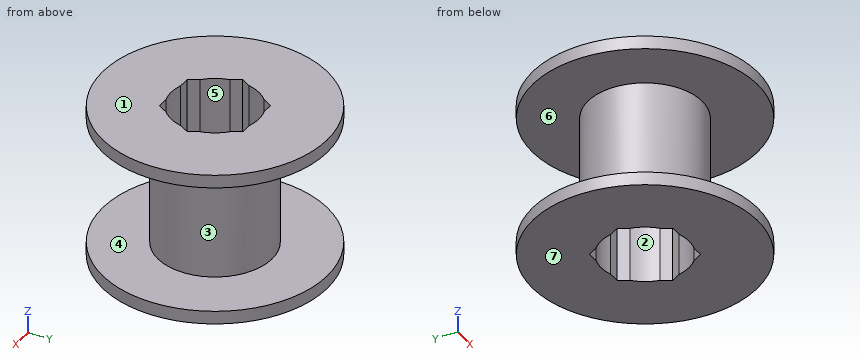
```python
from build123d import *

# Parameters (mm, degrees)
CUT_EXTRUDE1_DEPTH = 33.8


with BuildPart() as part:
    # Sketch1 → Revolve1 (revolve)
    with BuildSketch(Plane(origin=(0, 0, 0), x_dir=(0, 0, -1), z_dir=(1, 0, 0))):
        Polygon((-13.61, 23.9), (-13.61, 12.14), (13.61, 12.14), (13.61, 23.9), (16.4, 23.9), (16.4, 9.35), (-16.4, 9.35), (-16.4, 23.9), align=None)
    revolve(axis=Axis((0, 0, 33.448920863), (0, 0, -1)))

    # Sketch2 → Cut-Extrude1 (cut, through all)
    with BuildSketch(Plane.XY.offset(16.4)):
        Polygon((5.155737904, 8.93), (-5.155737904, 8.93), (-10.311475808, 0), (-5.155737904, -8.93), (5.155737904, -8.93), (10.311475808, 0), align=None)
    extrude(amount=-CUT_EXTRUDE1_DEPTH, mode=Mode.SUBTRACT)


solid = part.part
```
Geometry: final body of the model. Coordinates: model frame, mm. Face numbers are marked on the shaded views. A direction names the side the tool comes from. Coordinates: 2 decimals unless noted, no trailing zeros. Order: outer loops, then holes, each group sorted by start corner. A loop starts at its lowest first (then second) coordinate and runs counter-clockwise, first axis right, second up. Notation, with made-up numbers: (-17.5, 16) - (20.5, 16) arc R33 cw to (20.5, 47) - close; hole circle Ø7 at (49, 84.5). An arc over 180 degrees is marked (long way). Return JSON: item names as keys, results as strings. Group by question number.
1. Cut plane C-C (z = -3). Output: boundary loops of the cut face in (x, y), plus the area to 3 significant figures.
2. Set-up query: the marked faces 5, 6 and 7. Return all of +Z, -Z, +X, -X, +Y, -Y with unobstructed straight access to the full face (end or side cutting, diameter ignored); none if empty.
3. Pull-direction query (Z, two-part tool) for the marked faces 1, 2, 3 and 4; classes: pulls with the +Z half, pulls with the -Z half, needs draft (parallel to the pull), parting line crosses it, or undercut.
4. Cut plane A-A (x = 0). Output: boundary loops of the cut face in (y, z).
5. Cut plane B-B (y = 17.5). Output: boundary loops of the cut face in (x, z), plus the area to 3 significant figures.
6. Pin query (flat end, axial travel): pin 1 (1.5 mm diameter, centred on y = -6.5, z = -1.5, fed in from -X); pin 2 (4 mm diameter, centred on x = 16, z = 2, fed in from +Y); pin 3 (1.2 mm diameter, centred on x = 3.5, z = 6, fed in from +Y); pin 4 (4 mm diameter, centred on y = -1.5, z = -1.5, fed in from -X). Return the tip coordinate at first contact, or that it passes through.
7. Material intervals for line 1 along Z through (x, y) = (-13, 11.5); line 2 along Y through (x, z) = (7.5, -6.5); line 3 along Y through (x, z) = (-3, 11), sorted ascending. Write a range as [from, to].
8. Cut plane D-D (y = -20). Output: boundary loops of the cut face in (x, z), plus the area to 3 significant figures.
Resolved:
{
 "1": {"outline": "circle Ø24.28 at (0, 0); hole (-10.31, 0) - (-9.12, -2.07) arc R9.35 ccw to (-6.35, -6.86) - (-5.16, -8.93) - (-2.77, -8.93) arc R9.35 ccw to (2.77, -8.93) - (5.16, -8.93) - (6.35, -6.86) arc R9.35 ccw to (9.12, -2.07) - (10.31, 0) - (9.12, 2.07) arc R9.35 ccw to (6.35, 6.86) - (5.16, 8.93) - (2.77, 8.93) arc R9.35 ccw to (-2.77, 8.93) - (-5.16, 8.93) - (-6.35, 6.86) arc R9.35 ccw to (-9.12, 2.07) - close", "area": "177 mm²"},
 "2": {"face 5": "+Z, -Z", "face 6": "none", "face 7": "-Z, +X, -X, +Y, -Y"},
 "3": {"face 1": "pulls with the +Z half", "face 2": "needs draft", "face 3": "undercut", "face 4": "undercut"},
 "4": {"outline": "(-23.9, -16.4) - (-9.35, -16.4) - (-9.35, 16.4) - (-23.9, 16.4) - (-23.9, 13.61) - (-12.14, 13.61) - (-12.14, -13.61) - (-23.9, -13.61) - close; (9.35, -16.4) - (23.9, -16.4) - (23.9, -13.61) - (12.14, -13.61) - (12.14, 13.61) - (23.9, 13.61) - (23.9, 16.4) - (9.35, 16.4) - close"},
 "5": {"outline": "(-16.28, -16.4) - (16.28, -16.4) - (16.28, -13.61) - (-16.28, -13.61) - close; (-16.28, 13.61) - (16.28, 13.61) - (16.28, 16.4) - (-16.28, 16.4) - close", "area": "182 mm²"},
 "6": {"pin 1": "stops at x = -10.69", "pin 2": "passes through", "pin 3": "stops at y = 11.79", "pin 4": "stops at x = -12.14"},
 "7": {"line 1": "z = [-16.4, -13.61], [13.61, 16.4]", "line 2": "y = [-9.55, -5.58], [5.58, 9.55]", "line 3": "y = [-11.76, -8.93], [8.93, 11.76]"},
 "8": {"outline": "(-13.08, -16.4) - (13.08, -16.4) - (13.08, -13.61) - (-13.08, -13.61) - close; (-13.08, 13.61) - (13.08, 13.61) - (13.08, 16.4) - (-13.08, 16.4) - close", "area": "146 mm²"}
}
